```python
from build123d import *

# Parameters (mm, degrees)
SKETCH12_R         = 6.673371428
CORE_CYL_DEPTH     = 4.8
TOOTH_EX_DEPTH     = 4.8
CIRPATTERN1_COUNT  = 15
SKETCH13_W         = 4
SKETCH13_H         = 3.65
CUT_EXTRUDE1_DEPTH = 4


with BuildPart() as part:
    # Sketch12 → core_cyl (new body)
    with BuildSketch(Plane.XY):
        Circle(SKETCH12_R)
    extrude(amount=CORE_CYL_DEPTH)

    # tooth → tooth_ex (add)
    with BuildSketch(Plane.XY):
        with BuildLine():
            add(Edge.make_bspline(
                [(-0.089470773, 7.047126715), (-0.005108471, 7.588530401), (0.233889853, 8.063511638), (0.55714541, 8.481720874)],
                knots=[0, 0, 0, 0, 0.44996315, 0.44996315, 0.44996315, 0.44996315], degree=3))
            Line((-0.089470773, 7.047126715), (-0.128884861, 6.672126715))
            ThreePointArc((-0.128884861, 6.672126715), (0.69755726, 6.636814001), (1.513281564, 6.499528069))
            Line((1.513281564, 6.499528069), (1.552695653, 6.874528069))
            add(Edge.make_bspline(
                [(1.552695653, 6.874528069), (1.582741025, 7.421640695), (1.44771954, 7.935932997), (1.218478482, 8.412211968)],
                knots=[0, 0, 0, 0, 0.44996315, 0.44996315, 0.44996315, 0.44996315], degree=3))
            ThreePointArc((1.218478482, 8.412211968), (0.888491938, 8.453436111), (0.55714541, 8.481720874))
        make_face()
    tooth_ex = extrude(amount=TOOTH_EX_DEPTH)

    # CirPattern1: tooth_ex ×15 about axis
    cirpattern1_axis = Axis((0, 0, 0), (0, 0, 1))
    for i in range(1, CIRPATTERN1_COUNT):
        add(tooth_ex.rotate(cirpattern1_axis, i * 360 / CIRPATTERN1_COUNT))

    # Sketch13 → Cut-Extrude1 (cut)
    with BuildSketch(Plane.XY.offset(4.8)):
        with BuildLine():
            Line((-2, -1.825), (-2, 1.825))
            ThreePointArc((-2, 1.825), (-2.707512696, 0), (-2, -1.825))
        make_face()
        Rectangle(SKETCH13_W, SKETCH13_H)
        with BuildLine():
            ThreePointArc((2.707512696, 0), (2.524445523, 0.97867247), (2, 1.825))
            Line((2, 1.825), (2, -1.825))
            ThreePointArc((2, -1.825), (2.524445523, -0.97867247), (2.707512696, 0))
        make_face()
    extrude(amount=-CUT_EXTRUDE1_DEPTH, mode=Mode.SUBTRACT)


solid = part.part
```
Design review of the part built by this model. Coordinates are the model's own, in mm. A direction names the side the tool comes from. Coordinates: 2 decimals unless noted, no trailing zeros. Write each loop counter-clockwise with the first axis right and the second up, starting at its lowest first coordinate (ties: lowest second). Pieces come first, ordered by that corner, then holes.
1) Insertion check: pin 1 (1.1 mm diameter, centred on x = 1, y = 0, fed in from +Z). The pin has a flat end and moves straight along its axis. Give the tip position at first contact, or say it passes through.
2) To check wall thickness, follow L1, parallel to Y at x = -7.5, z = 3.9; L2, parallel to Y at x = -5.5, z = 1.45; L3, parallel to X at y = -7.25, z = 3.2. State the ranges of each line that lie inside material, in increasing order.
3) Mouldability with a two-part tool opening along X and no side actions: class faces 1 (the cylindrical face through (-6.53, -1.38, 2.37)), 2 (the flat face through (0, 0, 0.8)), 3 (the flat face through (0, 0, 0)), 4 (the cylindrical face through (6.673, -0.008, 2.366)) as +X half, -X half, draft (parallel to the pull), parting line (faces both ways), or undercut.
4) Add section A-A (x = 2.25). Write out the cut boundary in (y, z).
5) Machinability: for faces 5 (the flat face through (0, 2, 4.8)), 6 (the cylindrical face through (-0.69, 6.638, 2.366)), 7 (the cylindrical face through (4.459, -4.965, 2.366)), 8 (the flat face through (0, 1.825, 3)), which of the approach directions +Z, -Z, +X, -X, +Y, -Y give a long, thin tool a straight path to every point of the face, cutting with its end or side? Answer none if there is none.
Check result:
1. pin 1: stops at z = 0.8
2. L1: y = -3.77 to -2.66, -0.75 to 0.75, 2.66 to 3.77
2. L2: y = -6.48 to -4.93, -3.78 to 3.78, 4.93 to 6.48
2. L3: x = -3.04 to -1.53, -0.05 to 1.55, 3.53 to 4.44
3. face 1: -X half
3. face 2: undercut
3. face 3: draft
3. face 4: +X half
4. outline: (-6.28, 0) - (6.28, 0) - (6.28, 4.8) - (1.51, 4.8) - (1.51, 0.8) - (-1.51, 0.8) - (-1.51, 4.8) - (-6.28, 4.8) - close
5. face 5: +Z, +X, -X, +Y, -Y
5. face 6: +Z, -Z, +Y
5. face 7: +Z, -Z
5. face 8: +Z
